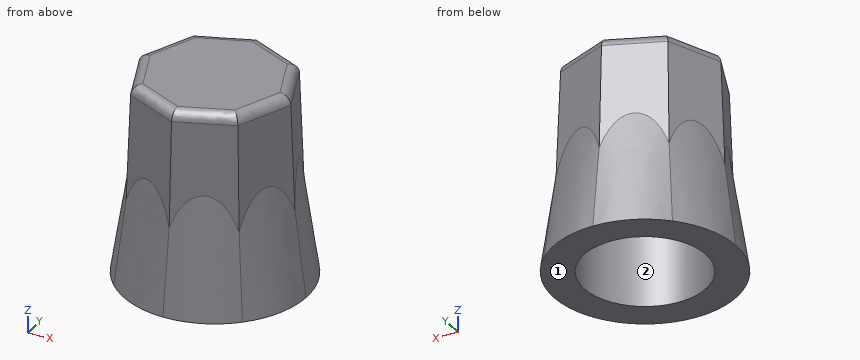
```python
from build123d import *

# Parameters (mm, degrees)
F5_R      = 15
F7_R      = 13.25
F9_R      = 2.5
F10_R     = 22.5
F12_R     = 15
F13_DEPTH = 45


with BuildPart() as f4:
    # F1 (on Top) → F4 section 0
    with BuildSketch(Plane.XY):
        Polygon((0, 20.5654518056), (-14.5419704299, 14.5419704299), (-20.5654518056, 0), (-14.5419704299, -14.5419704299), (0, -20.5654518056), (14.5419704299, -14.5419704299), (20.5654518056, 0), (14.5419704299, 14.5419704299), align=None)
    # F3 (on offset) → F4 section 1
    with BuildSketch(Plane.XY.offset(49)):
        Polygon((0, 18.671265455), (-13.2025784166, 13.2025784166), (-18.671265455, 0), (-13.2025784166, -13.2025784166), (0, -18.671265455), (13.2025784166, -13.2025784166), (18.671265455, 0), (13.2025784166, 13.2025784166), align=None)
    loft()

    # F5 (on Top) → F8 section 0
    with BuildSketch(Plane.XY):
        Circle(F5_R)
    # F7 (on offset) → F8 section 1
    with BuildSketch(Plane.XY.offset(45)):
        Circle(F7_R)
    loft(mode=Mode.SUBTRACT)

    # F9
    f9_edges = [f4.edges().sort_by_distance(p)[0] for p in [
        (-15.936922, -6.601289, 49),
        (-6.601289, -15.936922, 49),
        (6.601289, -15.936922, 49),
        (15.936922, -6.601289, 49),
        (15.936922, 6.601289, 49),
        (6.601289, 15.936922, 49),
        (-6.601289, 15.936922, 49),
        (-15.936922, 6.601289, 49),
    ]]
    fillet(f9_edges, radius=F9_R)

    # F10 (on Top) → F11 section 0
    with BuildSketch(Plane.XY):
        Circle(F10_R)
    # F4_face (on face) → F11 section 1
    with BuildSketch(Plane.XY.offset(49)):
        with BuildLine():
            add(Edge.make_bspline(
                [(-16.0602019121, 0), (-13.7082397957, -5.6781388396), (-11.3562776793, -11.3562776793)],
                knots=[0.9992107587, 0.9992107587, 0.9992107587, 13.2911571431, 13.2911571431, 13.2911571431], degree=2))
            add(Edge.make_bspline(
                [(-11.3562776793, -11.3562776793), (-5.6781388396, -13.7082397957), (0, -16.0602019121)],
                knots=[0.9992107587, 0.9992107587, 0.9992107587, 13.2911571431, 13.2911571431, 13.2911571431], degree=2))
            add(Edge.make_bspline(
                [(0, -16.0602019121), (5.6781388396, -13.7082397957), (11.3562776793, -11.3562776793)],
                knots=[0.9992107587, 0.9992107587, 0.9992107587, 13.2911571431, 13.2911571431, 13.2911571431], degree=2))
            add(Edge.make_bspline(
                [(11.3562776793, -11.3562776793), (13.7082397957, -5.6781388396), (16.0602019121, 0)],
                knots=[0.9992107587, 0.9992107587, 0.9992107587, 13.2911571431, 13.2911571431, 13.2911571431], degree=2))
            add(Edge.make_bspline(
                [(16.0602019121, 0), (13.7082397957, 5.6781388396), (11.3562776793, 11.3562776793)],
                knots=[0.9992107587, 0.9992107587, 0.9992107587, 13.2911571431, 13.2911571431, 13.2911571431], degree=2))
            add(Edge.make_bspline(
                [(11.3562776793, 11.3562776793), (5.6781388396, 13.7082397957), (0, 16.0602019121)],
                knots=[0.9992107587, 0.9992107587, 0.9992107587, 13.2911571431, 13.2911571431, 13.2911571431], degree=2))
            add(Edge.make_bspline(
                [(0, 16.0602019121), (-5.6781388396, 13.7082397957), (-11.3562776793, 11.3562776793)],
                knots=[0.9992107587, 0.9992107587, 0.9992107587, 13.2911571431, 13.2911571431, 13.2911571431], degree=2))
            add(Edge.make_bspline(
                [(-11.3562776793, 11.3562776793), (-13.7082397957, 5.6781388396), (-16.0602019121, 0)],
                knots=[0.9992107587, 0.9992107587, 0.9992107587, 13.2911571431, 13.2911571431, 13.2911571431], degree=2))
        make_face()
    loft()

    # F12 (on face) → F13 (cut)
    with BuildSketch(Plane(origin=(0, 0, 0), x_dir=(1, 0, 0), z_dir=(0, 0, -1))):
        Circle(F12_R)
    extrude(amount=-F13_DEPTH, mode=Mode.SUBTRACT)


solid = f4.part
```
CAD build for the part. Positions are in the model's coordinates, mm. Face numbers are marked on the shaded views. Round coordinates to 2 decimals unless told otherwise and drop trailing zeros. Return JSON: item names as keys, results as strings. Group by question number.
(1) Wall check: probe 1 along Y at (x, z) = (-12.5, 27); probe 2 along X at (y, z) = (13.5, 40); probe 3 along Z at (x, y) = (1, -1.5). Give the ranges that are in metal, low to high. Write a range as [from, to].
(2) Mould opens along X. For the marked faces 1 and 2 say: +X half, -X half, draft (parallel to the pull), parting line (faces both ways), or undercut.
(3) Drop flat-ended pins along their axis: P1, Ø6, axis at y = -0.5, z = 32, coming from the -X side; P2, Ø15, axis at x = -3, y = -5, coming from the -Z side; P3, Ø12, axis at y = 6.5, z = 38, coming from the -X side; P4, Ø1.5, axis at x = 2, y = -18, coming from the -Z side. Give the stop position or say it passes through.
Answer list:
{
 "1": {"probe 1": "[-14.34, -8.29], [8.29, 14.34]", "probe 2": "[-13.32, -6.54], [6.54, 13.32]", "probe 3": "[45, 49]"},
 "2": {"face 1": "draft", "face 2": "undercut"},
 "3": {"P1": "x = -19.44", "P2": "z = 45", "P3": "x = -18.9", "P4": "z = 0"}
}
